Job drawing, mm, ordinate dimensions from the low corner. One solid piece. Coordinates: 2 decimals unless noted, no trailing zeros. Write each loop counter-clockwise with the first axis right and the second up, starting at its lowest first coordinate (ties: lowest second). Pieces come first, ordered by that corner, then holes. Notation, with made-up numbers: (14.5, 59.25) - (18.5, 59.25) arc R5 ccw to (18.5, 68.25) - close; hole circle Ø3 at (-11.75, -4.5). An arc over 180 degrees is marked (long way). Use a Markdown table: item, result.
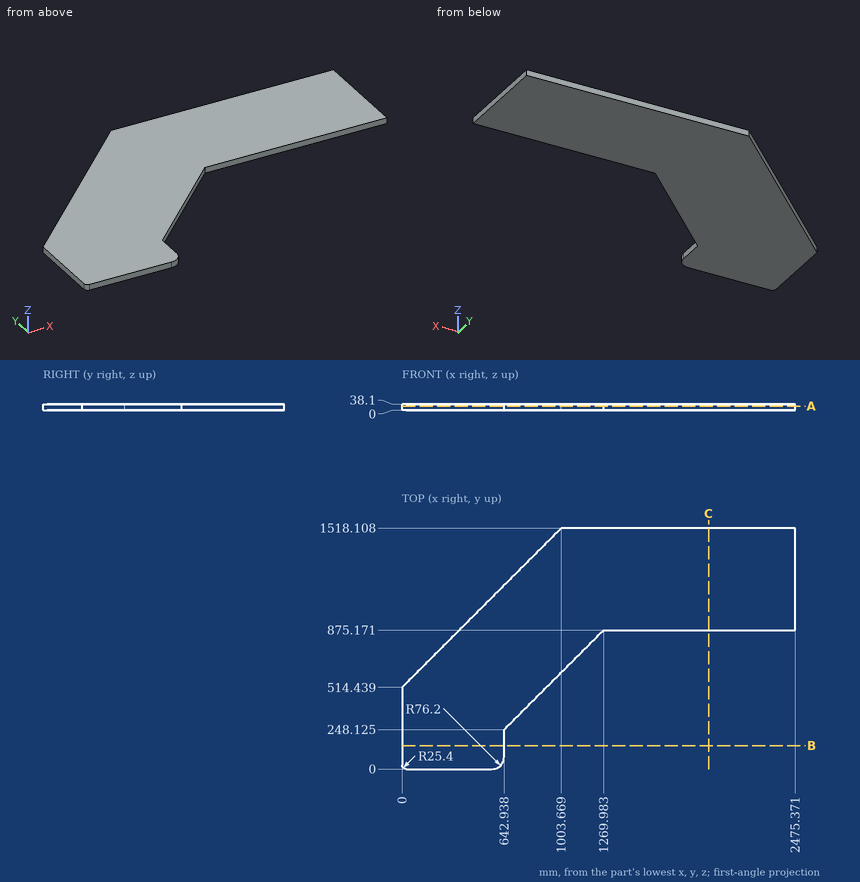
Item 1: Drop flat-ended pins along their axis: P1, Ø11.5, axis at y = 179.5, z = 23.5, coming from the +X side; P2, Ø8, axis at x = 1839, z = 17, coming from the -Y side; P3, Ø1, axis at x = 292, z = 8, coming from the -Y side; P4, Ø2, axis at y = 1226.5, z = 33, coming from the -X side. Give the stop position or say it passes through.
From the geometry:
| item | result |
|---|---|
| P1 | x = 642.94 |
| P2 | y = 875.17 |
| P3 | y = 0 |
| P4 | x = 711.06 |
Item 2: Drill centre lines: probe 1 along Y at (x, z) = (2081, 26); probe 2 along X at (y, z) = (244.5, 17.5); probe 3 along X at (y, z) = (382, 36.5) (1 decimal). Where is each one in solid material? Low to high.
From the geometry:
| item | result |
|---|---|
| probe 1 | 875.17 to 1518.11 |
| probe 2 | 0 to 642.94 |
| probe 3 | 0 to 776.8 |
Item 3: Band-saw the part on C-C, the plane x = 1931. Give the cut face in (y, z).
From the geometry:
| item | result |
|---|---|
| outline | (875.17, 0) - (1518.11, 0) - (1518.11, 38.1) - (875.17, 38.1) - close |
Item 4: Band-saw the part on A-A, the plane z = 24.5. Give the cut face in (x, y) (1 decimal), then the cut area to 3 significant figures.
From the geometry:
| item | result |
|---|---|
| outline | (0, 25.4) arc R25.4 ccw to (25.4, 0) - (566.7, 0) arc R76.2 ccw to (642.9, 76.2) - (642.9, 248.1) - (1270, 875.2) - (2475.4, 875.2) - (2475.4, 1518.1) - (1003.7, 1518.1) - (0, 514.4) - close |
| area | 1,850,000 mm^2 |
Item 5: Band-saw the part on B-B, the plane y = 148. Give the cut face in (x, z).
From the geometry:
| item | result |
|---|---|
| outline | (0, 0) - (642.94, 0) - (642.94, 38.1) - (0, 38.1) - close |
